Could you check a few things on this drawing? It's one solid part, dimensions in mm from its lowest x, y, z. Coordinates: 2 decimals unless noted, no trailing zeros. Write each loop counter-clockwise with the first axis right and the second up, starting at its lowest first coordinate (ties: lowest second). Pieces come first, ordered by that corner, then holes. Notation, with made-up numbers: (4.25, 32.5) - (15.25, 32.5) arc R33 ccw to (15.25, 61.5) - close; hole circle Ø2 at (68, 4.5). An arc over 180 degrees is marked (long way). Use one line per item in the form item = value. Start each with the question number.
(1) If we section it at C-C on x = 84.5: Please give me the cut outline in (y, z).
(2) If I drill on probe 1 along X at (y, z) = (2.2, 10); probe 2 along Z at (x, y) = (44, 0.55), over which ranges is the centre line in solid material (lowest first)? Write a range as from..to.
(3) For pin 1 Ø1.5 at (x, y) = (44.5, 1) entering from -Z, with a flat end and sliding along its axis, tell me the tip position at first contact or that it passes through.
(4) If we section it at B-B on y = 1.45: Please give me the cut outline in (x, z).
(5) If we section it at A-A on z = 15.5: Please give me the cut outline in (x, y), then the cut area to 3 significant figures.
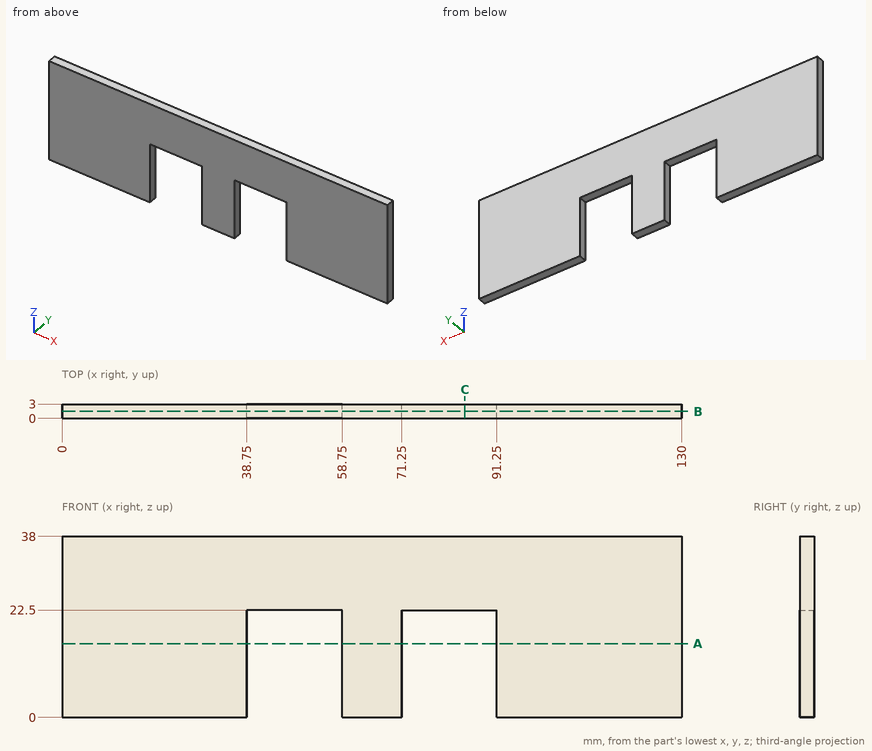
Reported:
q1.outline = (0, 22.5) - (3, 22.5) - (3, 38) - (0, 38) - close
q2.probe_1 = 0..38.75, 58.75..71.25, 91.25..130
q2.probe_2 = 22.5..38
q3.pin_1 = 22.5
q4.outline = (0, 0) - (38.75, 0) - (38.75, 22.5) - (58.75, 22.5) - (58.75, 0) - (71.25, 0) - (71.25, 22.5) - (91.25, 22.5) - (91.25, 0) - (130, 0) - (130, 38) - (0, 38) - close
q5.outline = (0, 0) - (38.75, 0) - (38.75, 3) - (0, 3) - close; (58.75, 0) - (71.25, 0) - (71.25, 3) - (58.75, 3) - close; (91.25, 0) - (130, 0) - (130, 3) - (91.25, 3) - close
q5.area = 270 mm2
